```python
from build123d import *

# Parameters (mm, degrees)
SKETCH1_W           = 25.1
SKETCH1_H           = 7
REVOLVE1_ANGLE      = 90
SKETCH2_W           = 7
SKETCH2_H           = 7
BOSS_EXTRUDE1_DEPTH = 10
SKETCH6_W           = 5
SKETCH6_H           = 7
BOSS_EXTRUDE2_DEPTH = 15
SKETCH7_W           = 5
SKETCH7_H           = 15
BOSS_EXTRUDE3_DEPTH = 6.5
SKETCH8_W           = 5
SKETCH8_H           = 15
BOSS_EXTRUDE4_DEPTH = 6.5
SKETCH10_R          = 2.1
CUT_EXTRUDE8_DEPTH  = 18.5
SKETCH12_R          = 1.1
CUT_EXTRUDE11_DEPTH = 10


with BuildPart() as part:
    # Sketch1 → Revolve1 (revolve)
    with BuildSketch(Plane(origin=(0, 0, 0), x_dir=(1, 0, 0), z_dir=(0, 1, 0))):
        with Locations((12.55, 3.5)):
            Rectangle(SKETCH1_W, SKETCH1_H)
    revolve(axis=Axis((0, 0, 0), (0, 0, 1)), revolution_arc=REVOLVE1_ANGLE)

    # Sketch2 → Boss-Extrude1 (add)
    with BuildSketch(Plane.ZY):
        with Locations((-3.5, 3.5)):
            Rectangle(SKETCH2_W, SKETCH2_H)
    extrude(amount=BOSS_EXTRUDE1_DEPTH)

    # Sketch6 → Boss-Extrude2 (add)
    with BuildSketch(Plane(origin=(0, 0, 0), x_dir=(-1, 0, 0), z_dir=(0, -1, 0))):
        with Locations((7.5, 3.5)):
            Rectangle(SKETCH6_W, SKETCH6_H)
    extrude(amount=BOSS_EXTRUDE2_DEPTH)

    # Sketch7 → Boss-Extrude3 (add)
    with BuildSketch(Plane.XY):
        with Locations((-7.5, -7.5)):
            Rectangle(SKETCH7_W, SKETCH7_H)
    extrude(amount=BOSS_EXTRUDE3_DEPTH)

    # Sketch8 → Boss-Extrude4 (add)
    with BuildSketch(Plane(origin=(0, 0, -7), x_dir=(-1, 0, 0), z_dir=(0, 0, -1))):
        with Locations((7.5, -7.5)):
            Rectangle(SKETCH8_W, SKETCH8_H)
    extrude(amount=BOSS_EXTRUDE4_DEPTH)

    # Sketch10 → Cut-Extrude8 (cut)
    with BuildSketch(Plane(origin=(-5, 0, 0), x_dir=(0, 0, -1), z_dir=(1, 0, 0))):
        with Locations((-1.216, -7.5)):
            Circle(SKETCH10_R)
        with Locations((7.882, -7.5)):
            Circle(SKETCH10_R)
    extrude(amount=-CUT_EXTRUDE8_DEPTH, mode=Mode.SUBTRACT)

    # Sketch12 → Cut-Extrude11 (cut)
    with BuildSketch(Plane.XY):
        with Locations((3, 3)):
            Circle(SKETCH12_R)
        with BuildLine():
            Line((3, 16.5), (3, 19.6))
            ThreePointArc((3, 19.6), (14.737972568, 14.737972568), (19.6, 3))
            Line((19.6, 3), (16.5, 3))
            ThreePointArc((16.5, 3), (12.545941546, 12.545941546), (3, 16.5))
        make_face()
    extrude(amount=-CUT_EXTRUDE11_DEPTH, mode=Mode.SUBTRACT)


solid = part.part
```
Check sheet for the modelled part. Datum: model origin and axes. Units: mm. A direction names the side the tool comes from. Round coordinates to 2 decimals unless told otherwise and drop trailing zeros. Loops run counter-clockwise (first coordinate to the right, second up) from the corner with the lowest first, then second, coordinate; pieces in that order, holes last. Notation, with made-up numbers: (-13.75, 1) - (25.25, 1) arc R33 ccw to (25.25, 33) - close; hole circle Ø11 at (27.25, -33.75). An arc over 180 degrees is marked (long way). Write item = value, one per line. Start each with the question number.
Q1. Release check for a two-part mould opening along Z. For faces 1 (the face through (-7.465, -5.418, 1.489)), 2 (the face through (-5, 7, -4)), 3 (the face through (8, 10, -7)) record: pulls with the +Z half, pulls with the -Z half, needs draft (parallel to the pull), parting line crosses it, or undercut.
Q2. Thickness scan on L1, parallel to Z at x = -7, y = -7; L2, parallel to X at y = -8.5, z = -11.25; L3, parallel to Z at x = 3.5, y = 22.5. Record the ranges inside material, lowest first.
Q3. Section check B-B (y = -7.5). Record the boundary of the cut face in (x, z).
Q4. Section check A-A (x = -6). Record the boundary of the cut face in (y, z).
Q5. Access from +Z, -Z, +X, -X, +Y, -Y to the whole of each face (thin tool, end or side, straight path). Record for faces 4 (the face through (-5, -8, -3)), 5 (the face through (-8, 0, 3)), 6 (the face through (12.65, 12.44, -3.45)), 7 (the face through (-7, 0, -10)).
Q6. Section check D-D (z = 0.5). Record the boundary of the cut face in (x, y).
Q7. Section check C-C (x = 8). Record the boundary of the cut face in (y, z).
Q8. Depth check by flat-ended pin: P1, Ø4.5, axis at y = -6, z = -0.5, coming from the +X side; P2, Ø5.5, axis at x = -6.5, z = -9, coming from the +Y side; P3, Ø12, axis at x = 19.5, y = 13.5, coming from the -Z side. Enter the tip coordinate at first touch or a pass-through.
Derived:
q1.face_1 = undercut
q1.face_2 = needs draft
q1.face_3 = pulls with the -Z half
q2.L1 = -13.5 to -9.92, -5.84 to -0.82, 3.26 to 6.5
q2.L2 = -10 to -5
q2.L3 = -7 to 0
q3.outline = (-10, -13.5) - (-5, -13.5) - (-5, -9.98) - (-10, -9.98) - close; (-10, -5.78) - (-5, -5.78) - (-5, -0.88) - (-10, -0.88) - close; (-10, 3.32) - (-5, 3.32) - (-5, 6.5) - (-10, 6.5) - close
q4.outline = (-15, -13.5) - (0, -13.5) - (0, -7) - (7, -7) - (7, 0) - (0, 0) - (0, 6.5) - (-15, 6.5) - close; hole circle Ø4.2 at (-7.5, -7.88); hole circle Ø4.2 at (-7.5, 1.22)
q5.face_4 = +Z, -Z, +X, -Y
q5.face_5 = +Z, +X, -X, +Y
q5.face_6 = +Z, -Z
q5.face_7 = -Z, +X, -X, +Y
q6.outline = (-10, -15) - (-5, -15) - (-5, -9.47) - (-10, -9.47) - close; (-10, -5.53) - (-5, -5.53) - (-5, 0) - (-10, 0) - close
q7.outline = (0, -7) - (15.54, -7) - (15.54, 0) - (0, 0) - close; (18.83, -7) - (23.79, -7) - (23.79, 0) - (18.83, 0) - close
q8.P1 = -5
q8.P2 = 7
q8.P3 = -7
